Work out the finished part from the listing and answer in its coordinate system (mm). Coordinates: 2 decimals unless noted, no trailing zeros. Write each loop counter-clockwise with the first axis right and the second up, starting at its lowest first coordinate (ties: lowest second). Pieces come first, ordered by that corner, then holes. Notation, with made-up numbers: M 42,24 L 101,24 A23 ccw 101,59 Z; hole C 61,-18.5 d10. An arc over 180 degrees is marked long. Use CSV: the item, a comma, the result in double quotes.
from build123d import *

# Parameters (mm, degrees)
BOSS_EXTRUDE1_DEPTH      = 3
BOSS_EXTRUDE1_DEPTH_BACK = 3
SKETCH2_R                = 4
CUT_EXTRUDE1_DEPTH       = 10


with BuildPart() as part:
    # Sketch1 → Boss-Extrude1 (new, two sides: drawn at the far end of the back side and taken through both)
    with BuildSketch(Plane.XY.offset(-BOSS_EXTRUDE1_DEPTH_BACK)):
        Polygon((8.571428571, -10), (23.571428571, -10), (4.821428571, 7.5), (-6.428571429, 7.5), (-6.428571429, -10), align=None)
    extrude(amount=BOSS_EXTRUDE1_DEPTH + BOSS_EXTRUDE1_DEPTH_BACK)

    # Sketch2 → Cut-Extrude1 (cut)
    with BuildSketch(Plane.XY.offset(3)):
        Circle(SKETCH2_R)
    extrude(amount=-CUT_EXTRUDE1_DEPTH, mode=Mode.SUBTRACT)


solid = part.part
Item 1: Consider probe 1 along Y at (x, z) = (0, -0.1); probe 2 along Y at (x, z) = (-2.5, -1.55); probe 3 along X at (y, z) = (-1.5, -1.2). Determine where each line is inside the solid, lowest interval first.
Answer:
probe 1,"y = -10 to -4, 4 to 7.5"
probe 2,"y = -10 to -3.12, 3.12 to 7.5"
probe 3,"x = -6.43 to -3.71, 3.71 to 14.46"
Item 2: The part is cut by section C-C (y = 0). Write down the section's boundary in (x, z).
Answer:
outline,"M -6.43,-3 L -4,-3 L -4,3 L -6.43,3 Z; M 4,-3 L 12.86,-3 L 12.86,3 L 4,3 Z"
Item 3: Given pin 1 (6.5 mm diameter, centred on x = 0, y = 0, fed in from +Z), flat-ended and moving along its own axis, determine where the tip first touches the part or whether it passes through.
Answer:
pin 1,"passes through"
Item 4: For a pull along X with two mould halves and no side action, classify faces 1 (the face through (-6.429, -1, 0)), 2 (the face through (-0.867, -3.905, 0.042)), 3 (the face through (5, -3, 3)) as released by +X, released by -X, zero draft, split by the parting line, or undercut.
Answer:
face 1,"released by -X"
face 2,"undercut"
face 3,"zero draft"
Item 5: The part is cut by section D-D (x = 12). Write down the section's boundary in (y, z).
Answer:
outline,"M -10,-3 L 0.8,-3 L 0.8,3 L -10,3 Z"
Item 6: The part is cut by section A-A (x = 0). Write down the section's boundary in (y, z).
Answer:
outline,"M -10,-3 L -4,-3 L -4,3 L -10,3 Z; M 4,-3 L 7.5,-3 L 7.5,3 L 4,3 Z"
Item 7: The part is cut by section B-B (z = 0.85). Write down the section's boundary in (x, y).
Answer:
outline,"M -6.43,-10 L 23.57,-10 L 4.82,7.5 L -6.43,7.5 Z; hole C 0,0 d8"
